Can you work these out from the model? Positions are in its coordinate system, mm. A direction names the side the tool comes from. Give positions to 0.01 mm unless a question says otherwise; leave off trailing zeros. Loops run counter-clockwise (first coordinate to the right, second up) from the corner with the lowest first, then second, coordinate; pieces in that order, holes last. Notation, with made-up numbers: (-18, -31) -> (28, -31) arc R33 ccw to (28, 4) -> close; hole circle Ø2 at (75.5, -9.75). An arc over 180 degrees is marked (long way). Use CSV: the item, a comma, the result in double quotes.
from build123d import *

# Parameters (mm, degrees)
SKETCH1_W           = 80
SKETCH1_H           = 12
BOSS_EXTRUDE1_DEPTH = 12
SKETCH2_R           = 2.1
CUT_EXTRUDE1_DEPTH  = 43.190046219
CUT_EXTRUDE8_DEPTH  = 0.2


with BuildPart() as part:
    # Sketch1 → Boss-Extrude1 (new body)
    with BuildSketch(Plane(origin=(0, 0, 0), x_dir=(1, 0, 0), z_dir=(0, 1, 0))):
        Rectangle(SKETCH1_W, SKETCH1_H)
    extrude(amount=BOSS_EXTRUDE1_DEPTH)

    # Sketch2 → Cut-Extrude1 (cut, through all)
    with BuildSketch(Plane(origin=(0, 12, 0), x_dir=(1, 0, 0), z_dir=(0, 1, 0))):
        with Locations(Location((35, 0, 0), (0, 0, 270))):
            Circle(SKETCH2_R)
        with Locations(Location((20, 0, 0), (0, 0, 270))):
            Circle(SKETCH2_R)
        with Locations(Location((-20, 0, 0), (0, 0, 90))):
            Circle(SKETCH2_R)
        with Locations(Location((-35, 0, 0), (0, 0, 90))):
            Circle(SKETCH2_R)
    extrude(amount=-CUT_EXTRUDE1_DEPTH, mode=Mode.SUBTRACT)

    # Sketch3 → Cut-Extrude8 (cut)
    with BuildSketch(Plane.ZY.offset(40)):
        Polygon((-3, 0), (0, 10.963509299), (3, 0), align=None)
    extrude(amount=-CUT_EXTRUDE8_DEPTH, mode=Mode.SUBTRACT)


solid = part.part
(1) Which directions (+Z, -Z, +X, -X, +Y, -Y) give clear straight access to the entire face, cutting with the end or side of a thin tool? Please do faces 4 (the face through (-39.8, 4, 0)), 5 (the face through (-40, 7.2, 1.4)).
Answer sheet:
face 4,"-X, -Y"
face 5,"+Z, -Z, -X, +Y, -Y"
(2) We'd pull the mould along Z, two halves only. Please class faces 1 (the face through (21.77, 6.08, 1.13)), 2 (the face through (-1, 6, 6)), 3 (the face through (-1, 0, 0)): released by +Z, released by -Z, zero draft, split by the parting line, or undercut.
Answer sheet:
face 1,"undercut"
face 2,"released by +Z"
face 3,"zero draft"
(3) If we section it at B-B, the plane y = 3.5: Write out the boundary of the cut face in (x, z), then the cut area to 3 significant figures.
Answer sheet:
outline,"(-40, -6) -> (40, -6) -> (40, 6) -> (-40, 6) -> (-40, 2.04) -> (-39.8, 2.04) -> (-39.8, -2.04) -> (-40, -2.04) -> close; hole circle Ø4.2 at (-35, 0); hole circle Ø4.2 at (-20, 0); hole circle Ø4.2 at (20, 0); hole circle Ø4.2 at (35, 0)"
area,"904 mm2"
(4) If I drill on L1, parallel to X at y = 4.75, z = 0; L2, parallel to Z at x = -35, y = 8.25; L3, parallel to X at y = 10.5, z = 0.25, over which ranges is the centre line in solid material (lowest first)? Write a range as from..to.
Answer sheet:
L1,"x = -39.8..-37.1, -32.9..-22.1, -17.9..17.9, 22.1..32.9, 37.1..40"
L2,"z = -6..-2.1, 2.1..6"
L3,"x = -40..-37.09, -32.91..-22.09, -17.91..17.91, 22.09..32.91, 37.09..40"
(5) Will this pin go through, and if not, where does the flat tip stop? pin 1 Ø3 at (y, z) = (8, 0) entering from -X.
Answer sheet:
pin 1,"stops at x = -40"
(6) If we section it at C-C, the plane y = 9.75: Write out the boundary of the cut face in (x, z).
Answer sheet:
outline,"(-40, -6) -> (40, -6) -> (40, 6) -> (-40, 6) -> (-40, 0.33) -> (-39.8, 0.33) -> (-39.8, -0.33) -> (-40, -0.33) -> close; hole circle Ø4.2 at (-35, 0); hole circle Ø4.2 at (-20, 0); hole circle Ø4.2 at (20, 0); hole circle Ø4.2 at (35, 0)"
(7) If we section it at A-A, the plane x = -20: Write out the boundary of the cut face in (y, z).
Answer sheet:
outline,"(0, -6) -> (12, -6) -> (12, -2.1) -> (0, -2.1) -> close; (0, 2.1) -> (12, 2.1) -> (12, 6) -> (0, 6) -> close"
